Input: part model. Units: mm. Frame: model coordinates. A direction names the side the tool comes from. Coordinates: 2 decimals unless noted, no trailing zeros. Order: outer loops, then holes, each group sorted by start corner. A loop starts at its lowest first (then second) coordinate and runs counter-clockwise, first axis right, second up.
from build123d import *

# Parameters (mm, degrees)
F0_R     = 3.175
F1_DEPTH = 3.175
F2_R     = 3.175
F3_DEPTH = 12.7
F4_R     = 3.175
F5_DEPTH = 3.175
F6_R     = 3.81
F7_DEPTH = 12.7


with BuildPart() as f1:
    # F0 (on Top) → F1 (new body)
    with BuildSketch(Plane.XY):
        Circle(F0_R)
    extrude(amount=F1_DEPTH)

    # F2 (on face) → F3 (join)
    with BuildSketch(Plane.XY.offset(3.175)):
        with BuildLine():
            ThreePointArc((7.62, -5.715), (9.0362084139, -3.0120694713), (9.525, 0))
            ThreePointArc((9.525, 0), (-3.0120694713, 9.0362084139), (-7.62, -5.715))
            Line((-7.62, -5.715), (7.62, -5.715))
        make_face()
        Circle(F2_R, mode=Mode.SUBTRACT)
        Circle(F2_R)
    extrude(amount=F3_DEPTH)

    # F4 (on face) → F5 (join)
    with BuildSketch(Plane.XY.offset(15.875)):
        Circle(F4_R)
    extrude(amount=F5_DEPTH)

    # F6 (on face) → F7 (cut)
    with BuildSketch(Plane.XZ.offset(5.715)):
        with Locations((0, 9.525)):
            Circle(F6_R)
    extrude(amount=-F7_DEPTH, mode=Mode.SUBTRACT)


solid = f1.part
Item 1: Cut plane A-A on x = 0. Return loops of the section in (y, z) (3 decimals), then the cut area to 3 significant figures.
Response values:
outline: (-5.715, 3.175) - (-3.175, 3.175) - (-3.175, 0) - (3.175, 0) - (3.175, 3.175) - (9.525, 3.175) - (9.525, 15.875) - (3.175, 15.875) - (3.175, 19.05) - (-3.175, 19.05) - (-3.175, 15.875) - (-5.715, 15.875) - (-5.715, 13.335) - (6.985, 13.335) - (6.985, 5.715) - (-5.715, 5.715) - close
area: 137 mm2
Item 2: Cut plane D-D on y = -0.5. Return loops of the section in (x, z) (3 decimals), then the cut area to 3 significant figures.
Response values:
outline: (-9.512, 3.175) - (-3.135, 3.175) - (-3.135, 0) - (3.135, 0) - (3.135, 3.175) - (9.512, 3.175) - (9.512, 15.875) - (3.135, 15.875) - (3.135, 19.05) - (-3.135, 19.05) - (-3.135, 15.875) - (-9.512, 15.875) - close; hole circle Ø7.62 at (0, 9.525)
area: 236 mm2
Item 3: Draft query along Z for faces 1 (the face through (0, 4, 3.175)), 2 (the face through (-0.8, 0.5, 5.8)), 3 (the face through (-0.69, -3.1, 1.57)). Return one class per face: pulls with the +Z half, pulls with the -Z half, needs draft (parallel to the pull), parting line crosses it, or undercut.
Response values:
face 1: pulls with the -Z half
face 2: undercut
face 3: needs draft
Item 4: Access query for faces 4 (the face through (-0.69, -3.1, 17.44)), 5 (the face through (0, 0, 19.05)), 6 (the face through (0, 6.985, 10)). Directions: +Z, -Z, +X, -X, +Y, -Y. A direction counts if a zero-diameter tool reaches every point of the face in a straight line with its end or side. Return the directions, or none.
Response values:
face 4: +Z
face 5: +Z, +X, -X, +Y, -Y
face 6: -Y
Item 5: Cut plane C-C on z = 12.25. Return loops of the section in (x, y) (3 decimals), then the cut area to 3 significant figures.
Response values:
outline: (-7.62, -5.715) - (-2.663, -5.715) - (-2.663, 6.985) - (2.663, 6.985) - (2.663, -5.715) - (7.62, -5.715) arc R9.525 ccw (long way) to start
area: 177 mm2
Item 6: Ray query, probe 1 along Z at (x, y) = (0, -1.75) (3 decimals); probe 2 along Z at (x, y) = (4.5, 3) (3 decimals); probe 3 along X at (y, z) = (-0.25, 9). Return the intervals inside material, ascending.
Response values:
probe 1: z = 0 to 5.715, 13.335 to 19.05
probe 2: z = 3.175 to 15.875
probe 3: x = -9.52 to -3.77, 3.77 to 9.52
Item 7: Pin query (flat end, axial travel): pin 1 Ø1.5 at (y, z) = (7, 4.5) entering from -X; pin 2 Ø5 at (x, y) = (4, 6.5) entering from +Z (3 decimals); pin 3 Ø5 at (y, z) = (4.5, 5) entering from -X. Return the tip coordinate at first contact, or that it passes through.
Response values:
pin 1: stops at x = -7.19
pin 2: stops at z = 15.875
pin 3: stops at x = -9.31
Item 8: Cut plane B-B on y = 2. Return loops of the section in (x, z) (3 decimals).
Response values:
outline: (-9.313, 3.175) - (-2.466, 3.175) - (-2.466, 0) - (2.466, 0) - (2.466, 3.175) - (9.313, 3.175) - (9.313, 15.875) - (2.466, 15.875) - (2.466, 19.05) - (-2.466, 19.05) - (-2.466, 15.875) - (-9.313, 15.875) - close; hole circle Ø7.62 at (0, 9.525)
